Design review of the part shown in the three views and the two pictorial views. Dimensions are in mm from the part's minimum x, y and z. Round coordinates to 2 decimals unless told otherwise and drop trailing zeros. Write each loop counter-clockwise with the first axis right and the second up, starting at its lowest first coordinate (ties: lowest second). Pieces come first, ordered by that corner, then holes. Notation, with made-up numbers: (-34.75, 58) - (-6.75, 58) arc R28 ccw to (-6.75, 80) - close; hole circle Ø7 at (-11, 63). An arc over 180 degrees is marked (long way). One line per item, written item: value. Start each with the question number.
Q1. Add section C-C on x = 7.75. Write out the cut boundary in (y, z) (1 decimal).
Q2. For probe 1 along X at (y, z) = (23, 65) (1 decimal); probe 2 along X at (y, z) = (18.75, 36) (1 decimal), list the stretches that pass through material, from the lowest coordinate up.
Q3. Clearance check with a flat-ended pin moving along its axis: pin 1 Ø5 at (x, z) = (13, 61) entering from -Y. State where the tip first meets the part, or that it passes through.
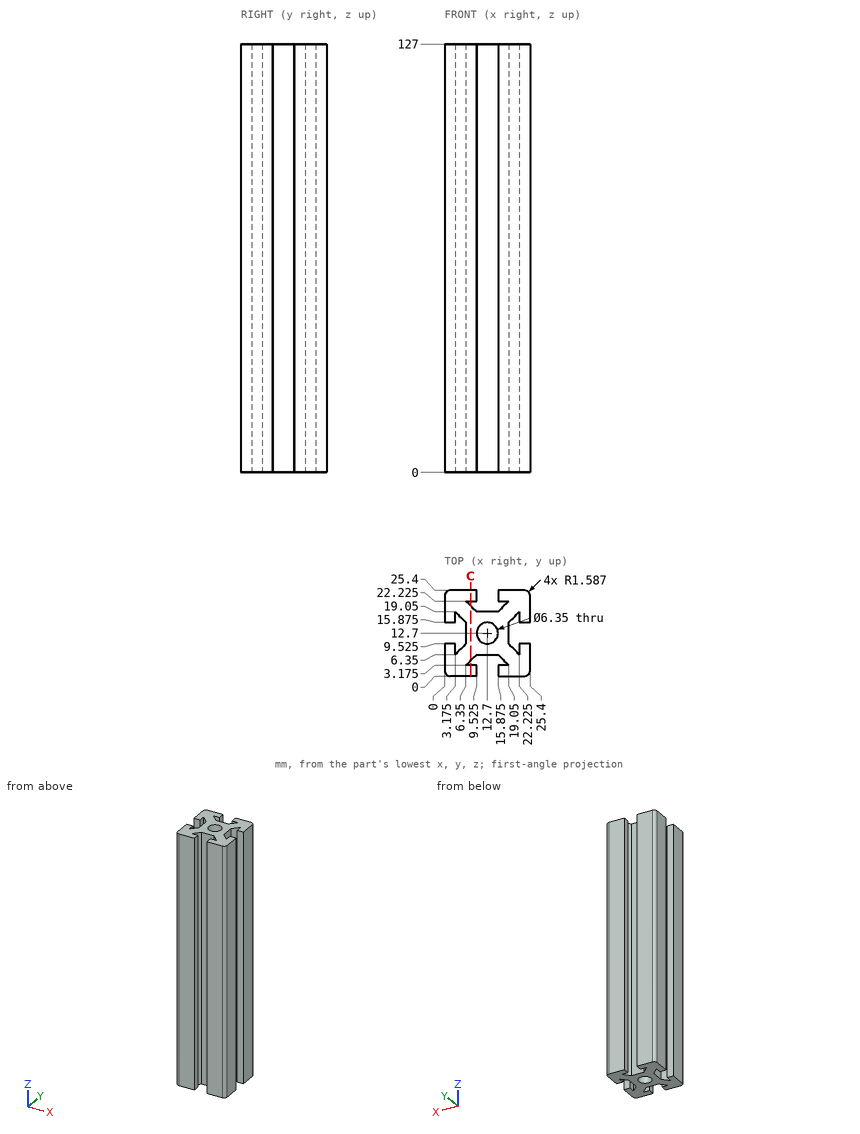
Result set:
1. outline: (0, 0) - (3.2, 0) - (3.2, 127) - (0, 127) - close; (4.6, 0) - (20.8, 0) - (20.8, 127) - (4.6, 127) - close; (22.2, 0) - (25.4, 0) - (25.4, 127) - (22.2, 127) - close
2. probe 1: x = 0 to 9.5, 15.9 to 25.4
2. probe 2: x = 0 to 3.2, 3.5 to 21.9, 22.2 to 25.4
3. pin 1: stops at y = 6.35
